Here's how the part is built. I have some questions about the finished solid (model axes, mm). A direction names the side the tool comes from. Give positions to 0.01 mm unless a question says otherwise; leave off trailing zeros. Write each loop counter-clockwise with the first axis right and the second up, starting at its lowest first coordinate (ties: lowest second). Pieces come first, ordered by that corner, then holes. Notation, with made-up numbers: M -36.5,-15 L 13.5,-15 A26 cw 13.5,7 Z; hole C 24.25,-2 d4. An arc over 180 degrees is marked long. Answer as CSV lines item,"result". Start each with the question number.
Q1. If I drill on line 1 along Z through (x, y) = (0, -2.1); line 2 along X through (y, z) = (80, 0); line 3 along Y through (x, z) = (-15, -28), over which ranges is the centre line in solid material (lowest first)?
Q2. For pin 1 (3 mm diameter, centred on x = -25.5, z = 21.5, fed in from +Y); pin 2 (3 mm diameter, centred on x = 8, y = 80.5, fed in from +Z); pin 3 (2.5 mm diameter, centred on x = -4, z = -29, fed in from +Y), each with a flat end and sliding along its axis, tell me the tip position at first contact or that it passes through.
Q3. Thinking about a two-plate mould opening in Y: for faces 4 (the flat face through (0, 0, 31)), 5 (the flat face through (-24, 0, 24)), 6 (the flat face through (0.2, -4, 30.3)), 7 (the flat face through (-24, -3.5, 24)), which applies, +Y half, -Y half, draft (parallel to the pull), parting line (faces both ways), or undercut?
Q4. Suppose I cut it at A-A (z = 0). Write out the boundary of the cut face in (x, y), then the cut area to 3 significant figures.
Q5. On a 3-axis mill with a long thin cutter (end or side, diameter ignored), from which of +Z, -Z, +X, -X, +Y, -Y can I reach the whole of each face in a straight line? I mean faces 1 (the flat face through (-24, -3.5, -24)), 2 (the cylindrical face through (19.55, -1.73, -27.23)), 3 (the flat face through (0.1, 0, -30.3)). Say none if no direction works.
Q6. Suppose I cut it at C-C (y = 5.5). Write out the boundary of the cut face in (x, z).
Q7. Suppose I cut it at D-D (z = 7.5). Write out the boundary of the cut face in (x, y), then the cut area to 3 significant figures.
Q8. Suppose I cut it at B-B (x = 17). Write out the boundary of the cut face in (y, z), then the cut area to 3 significant figures.
Autodesk Inventor part; units mm, degrees
ref_plane "YZ Plane" through (0, 0, 0) normal (1, 0, 0) x (0, 1, 0)
ref_plane "XZ Plane" through (0, 0, 0) normal (0, 1, 0) x (-1, 0, 0)
ref_plane "XY Plane" through (0, 0, 0) normal (0, 0, 1) x (1, 0, 0)
sketch "Sketch1" plane through (0, 0, 0) normal (0, 1, 0) x (-1, 0, 0)
  circle A0 centre (0, 0) radius 32
  circle A1 centre (0, 0) radius 34
  circle A2 centre (0, 0) radius 30
  line L0 (0, 34) -> (0, 32)
  line L1 (0, -32) -> (0, -34)
  dimension "d0" = 64
  dimension "d1" = 2
  dimension "d2" = 2
extrude "Extrusion1" add sketch "Sketch1" along normal blind 100 contours A0 L1 A1 L0 picked at (-2.7122, -33.004)
sketch "Sketch2" plane through (0, 0, 0) normal (0, 1, 0) x (-1, 0, 0)
  circle A0 centre (0, 0) radius 30
  circle A1 centre (0, 0) radius 32
extrude "Extrusion2" add sketch "Sketch2" against normal blind 4
sketch "Sketch3" plane through (0, 0, 0) normal (0, 1, 0) x (-1, 0, 0)
  circle A0 centre (0, 0) radius 37
  arc A1 (0, -32) -> (0, 32) centre (0, 0) ccw
  circle A2 centre (0, 0) radius 30
  circle A3 centre (0, 0) radius 32
  point P0 (0, 32)
  dimension "d7" = 74
extrude "Extrusion3" add sketch "Sketch3" along normal mid plane 8 contours A0
sketch "Sketch4" plane through (0, 0, 0) normal (0, 1, 0) x (-1, 0, 0)
  circle A0 centre (24, 24) radius 5.5
  circle A1 centre (0, 0) radius 30
  line L0 (48.965, 0) -> (-22.6719, 0) construction
  circle A2 centre (0, 0) radius 37
  line L1 (24, 24) -> (0, 0) construction
  circle A3 centre (-24, 24) radius 5.5
  circle A4 centre (-24, -24) radius 5.5
  circle A5 centre (24, -24) radius 5.5
  point P0 (22.5777, 29.3129)
  point P1 (29.3129, 22.5777)
  dimension "d10" = 11
  dimension "d11" = 45
  dimension "d16" = 24
  dimension "d19" = 360
extrude "Extrusion6" cut sketch "Sketch4" against normal blind 3.5 contours A0 A2 | A2 A0 A1 | A1 A0 | A3 A1 A2 | A2 A3 | A3 A1 | A5 A2 | A2 A5 A1 | A4 A1 A2 | A2 A4 | A1 A5 | A4 A1
properties part number "Kessil holder"
Resolved:
1,line 1,"-37 to -30, 30 to 37"
1,line 2,"32 to 34"
1,line 3,"-4 to 0"
2,pin 1,"y = 4"
2,pin 2,"z = 33.37"
2,pin 3,"y = 0"
3,face 4,"+Y half"
3,face 5,"undercut"
3,face 6,"-Y half"
3,face 7,"undercut"
4,outline,"M -37,-4 L -30,-4 L -30,0 L -32,0 L -32,4 L -37,4 Z; M 30,-4 L 37,-4 L 37,4 L 34,4 L 34,100 L 32,100 L 32,0 L 30,0 Z"
4,area,"288 mm^2"
5,face 1,"none"
5,face 2,"+X"
5,face 3,"+Y"
6,outline,"M 0,-34 A34 ccw 0,34 L 0,32 A32 cw 0,-32 Z"
7,outline,"M -36.23,-4 L -29.05,-4 L -29.05,0 L -31.11,0 L -31.11,4 L -36.23,4 Z; M 29.05,-4 L 36.23,-4 L 36.23,4 L 33.16,4 L 33.16,100 L 31.11,100 L 31.11,0 L 29.05,0 Z"
7,area,"296 mm^2"
8,outline,"M -4,-32.86 L 4,-32.86 L 4,-29.44 L 100,-29.44 L 100,-27.11 L 0,-27.11 L 0,-24.72 L -4,-24.72 Z; M -4,24.72 L 0,24.72 L 0,27.11 L 100,27.11 L 100,29.44 L 4,29.44 L 4,32.86 L -4,32.86 Z"
8,area,"559 mm^2"
